from build123d import *

# Parameters (mm, degrees)
SKETCH_2_R          = 1.5
CUT_EXTRUDE_1_DEPTH = 5
SKETCH_3_W          = 5.127083255
SKETCH_3_H          = 1.657522806
CUT_EXTRUDE_2_DEPTH = 8


with BuildPart() as part:
    # 草图1 → 旋转1 (revolve)
    with BuildSketch(Plane.XY, mode=Mode.PRIVATE) as revolve_1_sk:
        Polygon((30, 17.5), (30, 12.2), (30, 3.25), (32, 3.25), (32, 0), (30.858335085, 0), (0, 0), (-19.941664915, 0), (-22.441664915, 0), (-31.441664915, 0), (-31.441664915, 2), (-22.441664915, 2), (-22.5, 2.168145965), (-22.5, 3.5), (-20, 3.5), (-20, 18.5), (0, 18.5), (0, 17.5), align=None)
    revolve(revolve_1_sk.sketch.rotate(Axis((-72.034969576, 0, 0), (1, 0, 0)), 90), axis=Axis((-72.034969576, 0, 0), (1, 0, 0)))

    # 草图2 → 切除-拉伸1 (cut)
    with BuildSketch(Plane.ZY.offset(20)):
        with Locations((15.5, 0)):
            Circle(SKETCH_2_R)
        with Locations((7.75, -13.423393759)):
            Circle(SKETCH_2_R)
        with Locations((-7.75, -13.423393759)):
            Circle(SKETCH_2_R)
        with Locations((-15.5, 0)):
            Circle(SKETCH_2_R)
        with Locations((-7.75, 13.423393759)):
            Circle(SKETCH_2_R)
        with Locations((7.75, 13.423393759)):
            Circle(SKETCH_2_R)
    extrude(amount=-CUT_EXTRUDE_1_DEPTH, mode=Mode.SUBTRACT)

    # 草图3 → 切除-拉伸2 (cut)
    with BuildSketch(Plane.ZY.offset(31.441664915)):
        with Locations((0.013848215, 2.328761403)):
            Rectangle(SKETCH_3_W, SKETCH_3_H)
    extrude(amount=-CUT_EXTRUDE_2_DEPTH, mode=Mode.SUBTRACT)


solid = part.part
The model under review builds one solid part; all positions refer to its coordinate system, in mm. A direction names the side the tool comes from. Round coordinates to 2 decimals unless told otherwise and drop trailing zeros. Loops run counter-clockwise (first coordinate to the right, second up) from the corner with the lowest first, then second, coordinate; pieces in that order, holes last. Notation, with made-up numbers: M -6.5,69 L 45.5,69 A20 cw 45.5,88 Z; hole C 3.25,36 d6. An arc over 180 degrees is marked long. Answer as a JSON object with one key per item and string values.
Item 1: For line 1 along Y through (x, z) = (-18.2, 7.75); line 2 along Z through (x, y) = (-17.5, 12.5); line 3 along X through (y, z) = (-9, 16), list the stretches that pass through material, from the lowest coordinate up.
Check sheet entries:
{"line 1": "-16.8 to -14.92, -11.92 to 11.92, 14.92 to 16.8", "line 2": "-13.64 to -8.93, -6.57 to 6.57, 8.93 to 13.64", "line 3": "-20 to 0"}
Item 2: Clearance check with flat-ended pins moving along their axes: P1, Ø5, axis at y = -13.42, z = 7.75, coming from the -X side; P2, Ø1.5, axis at x = -20, z = 10, coming from the +Y side; P3, Ø8, axis at x = -11, z = -11.5, coming from the +Y side; P4, Ø18.5, axis at y = 4, z = -2, coming from the -X side. State where each tip first meets the part, or that it passes through.
Check sheet entries:
{"P1": "x = -20", "P2": "y = 16.02", "P3": "y = 16.91", "P4": "x = -31.44"}
Item 3: The part is to be moulded in two halves that separate along Y. For faces 5 (the face through (-22.5, 2, 2)), 6 (the face through (31.014, 1.978, -2.579)), 7 (the face through (-15, 0, -16)), say which applies: +Y half, -Y half, draft (parallel to the pull), parting line (faces both ways), or undercut.
Check sheet entries:
{"face 5": "draft", "face 6": "parting line", "face 7": "undercut"}
Item 4: We need section B-B, the plane z = 0. State the section outline as (x, y) points, and give its area (3 significant figures).
Check sheet entries:
{"outline": "M -31.44,-2 L -22.44,-2 L -22.5,-2.17 L -22.5,-3.5 L -20,-3.5 L -20,-18.5 L 0,-18.5 L 0,-17.5 L 30,-17.5 L 30,-3.25 L 32,-3.25 L 32,3.25 L 30,3.25 L 30,17.5 L 0,17.5 L 0,18.5 L -20,18.5 L -20,3.5 L -22.5,3.5 L -22.5,2.17 L -22.44,2 L -23.44,2 L -23.44,1.5 L -31.44,1.5 Z", "area": "1,850 mm2"}
Item 5: We need section C-C, the plane x = 2. State the section outline as (y, z) points, and give its area (3 significant figures).
Check sheet entries:
{"outline": "C 0,0 d35", "area": "962 mm2"}
Item 6: We need section D-D, the plane z = 10. State the section outline as (x, y) points, and give its area (3 significant figures).
Check sheet entries:
{"outline": "M -20,-15.56 L 0,-15.56 L 0,-14.36 L 30,-14.36 L 30,14.36 L 0,14.36 L 0,15.56 L -20,15.56 Z", "area": "1,480 mm2"}
Item 7: Tool access review of faces 1 (the face through (0, 14, -11)), 2 (the face through (-9.86, 16.41, 8.54)), 3 (the face through (-27, 1.5, 0)), 4 (the face through (-17.535, -12.41, -8.856)): name each direction out of +Z, -Z, +X, -X, +Y, -Y from which nothing blocks a thin tool from reaching the whole face with its end or side.
Check sheet entries:
{"face 1": "+X", "face 2": "+X, -X", "face 3": "+Z, -Z, -X, +Y", "face 4": "-X"}
